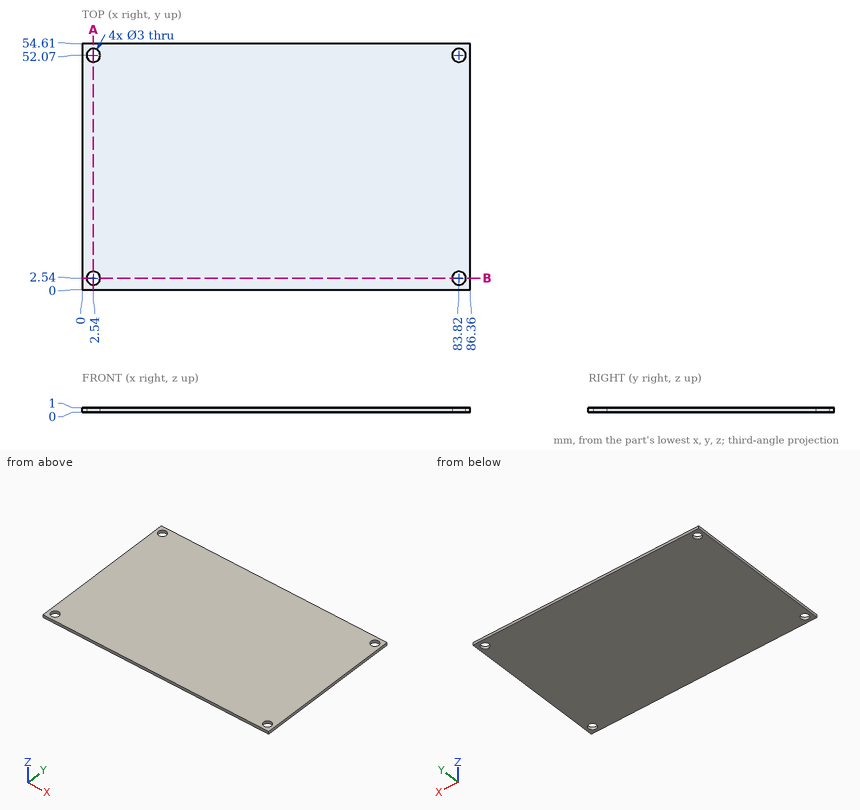
Source: three-view drawing plus pictorial views. Frame: mm from the lowest corner of the part. Give positions to 0.01 mm unless a question says otherwise; leave off trailing zeros. Write each loop counter-clockwise with the first axis right and the second up, starting at its lowest first coordinate (ties: lowest second). Pieces come first, ordered by that corner, then holes. Notation, with made-up numbers: (-37.5, 13.5) -> (16.5, 13.5) arc R18 ccw to (16.5, 17.5) -> close; hole circle Ø2 at (-16.5, 65.5). An arc over 180 degrees is marked (long way). Write item = value, one per line.
Q1. Cut plane A-A on x = 2.54. Return loops of the section in (y, z).
Here are the results:
outline = (0, 0) -> (1.04, 0) -> (1.04, 1) -> (0, 1) -> close; (4.04, 0) -> (50.57, 0) -> (50.57, 1) -> (4.04, 1) -> close; (53.57, 0) -> (54.61, 0) -> (54.61, 1) -> (53.57, 1) -> close
Q2. First-contact query: pin 1 (1.8 mm diameter, centred on x = 83.82, y = 2.54, fed in from +Z). Flat tip, straight axial feed; report the tip coordinate or a pass-through.
Here are the results:
pin_1 = through
Q3. Line query: line 1 (Y direction, x = 83.82, z = 0.45); line 2 (X direction, y = 52, z = 0.65). Output: solid intervals per line, ascending. Write a range as from..to.
Here are the results:
line_1 = 0..1.04, 4.04..50.57, 53.57..54.61
line_2 = 0..1.04, 4.04..82.32, 85.32..86.36
Q4. Cut plane B-B on y = 2.54. Return loops of the section in (x, z), then the cut area to 3 significant figures.
Here are the results:
outline = (0, 0) -> (1.04, 0) -> (1.04, 1) -> (0, 1) -> close; (4.04, 0) -> (82.32, 0) -> (82.32, 1) -> (4.04, 1) -> close; (85.32, 0) -> (86.36, 0) -> (86.36, 1) -> (85.32, 1) -> close
area = 80.4 mm²
